Model file for the job. Use its own axes, mm. Face numbers are marked on the shaded views. Coordinates: 2 decimals unless noted, no trailing zeros. Write each loop counter-clockwise with the first axis right and the second up, starting at its lowest first coordinate (ties: lowest second). Pieces come first, ordered by that corner, then holes. Notation, with made-up numbers: M -37.75,13.5 L -11.75,13.5 A7 ccw -11.75,17.5 Z; hole C -7.75,39.25 d4. An arc over 180 degrees is marked long. Answer in a Markdown table with one row per item. Add a question column.
```python
from build123d import *
from build123d.topology import SkipClean

# Parameters (mm, degrees)
CUT_EXTRUDE_START        = -10
CUT_EXTRUDE_1_DEPTH      = 10
EXTRUDE_1_DEPTH          = 6
PATTERN_CIRCULAR_1_COUNT = 3
SKETCH_4_R               = 42.404307435
SKETCH_4_R_2             = 25.5
CUT_EXTRUDE_2_DEPTH      = 9.5
CHAMFER_START            = 14
CHAMFER_1_DEPTH          = 6


with BuildPart() as part:
    # Эскиз1 → Повернуть1 (revolve)
    with BuildSketch(Plane.XY, mode=Mode.PRIVATE) as revolve_1_sk:
        Polygon((-24, 0), (-24, 4.5), (-26, 4.5), (-26, 9.5), (-19, 9.5), (-19, 22), (-24, 22), (-24, 12.5), (-29, 12.5), (-29, 0), align=None)
    revolve(revolve_1_sk.sketch.rotate(Axis((0, 0, 0), (0, -1, 0)), 270), axis=Axis((0, 0, 0), (0, -1, 0)))

    # Эскиз2 → Вырез-Вытянуть1 (cut)
    with SkipClean():  # the faces are left unmerged after this step: merging them gives an invalid solid
        with BuildSketch(Plane(origin=(0, 0, 0), x_dir=(-1, 0, 0), z_dir=(0, -1, 0)).offset(CUT_EXTRUDE_START)):
            with BuildLine():
                ThreePointArc((24, 0), (17.8818714, -16.007456864), (2.646777063, -23.85360709))
                Line((2.646777063, -23.85360709), (5, -25.514701644))
                ThreePointArc((5, -25.514701644), (20.0748599, -16.522711642), (26, 0))
                ThreePointArc((26, 0), (25.646694472, 4.271658071), (24.596379794, 8.427223803))
                Line((24.596379794, 8.427223803), (21.981218243, 9.63462737))
                ThreePointArc((21.981218243, 9.63462737), (23.489883331, 4.921928594), (24, 0))
            make_face()
            with BuildLine():
                Line((-5, -25.514701644), (-2.646777063, -23.85360709))
                ThreePointArc((-2.646777063, -23.85360709), (-20.784609691, -12), (-21.981218243, 9.63462737))
                Line((-21.981218243, 9.63462737), (-24.596379794, 8.427223803))
                ThreePointArc((-24.596379794, 8.427223803), (-22.516660498, -13), (-5, -25.514701644))
            make_face()
            with BuildLine():
                Line((-19.596379794, 17.087477841), (-19.33444118, 14.218979719))
                ThreePointArc((-19.33444118, 14.218979719), (0, 24), (19.33444118, 14.218979719))
                Line((19.33444118, 14.218979719), (19.596379794, 17.087477841))
                ThreePointArc((19.596379794, 17.087477841), (0, 26), (-19.596379794, 17.087477841))
            make_face()
        extrude(amount=CUT_EXTRUDE_1_DEPTH, mode=Mode.SUBTRACT)

    # Эскиз3 → Бобышка-Вытянуть1 (add)
    with SkipClean():  # the faces are left unmerged after this step: merging them gives an invalid solid
        with BuildSketch(Plane(origin=(25.5, 0, 0), x_dir=(0, 0, -1), z_dir=(1, 0, 0))):
            Polygon((-11.5, 20), (11.5, 20), (11.5, 17), (-11.5, 15), align=None)
        extrude_1 = extrude(amount=-EXTRUDE_1_DEPTH)

    # Круговой массив1: Бобышка-Вытянуть1 ×3 about axis
    with SkipClean():  # the faces are left unmerged after this step: merging them gives an invalid solid
        pattern_circular_1_axis = Axis((0, 0, 0), (0, 1, 0))
        for i in range(1, PATTERN_CIRCULAR_1_COUNT):
            add(extrude_1.rotate(pattern_circular_1_axis, i * 360 / PATTERN_CIRCULAR_1_COUNT))

    # Эскиз4 → Вырез-Вытянуть2 (cut)
    with SkipClean():  # the faces are left unmerged after this step: merging them gives an invalid solid
        with BuildSketch(Plane(origin=(0, 22, 0), x_dir=(1, 0, 0), z_dir=(0, 1, 0))):
            Circle(SKETCH_4_R)
            Circle(SKETCH_4_R_2, mode=Mode.SUBTRACT)
        extrude(amount=-CUT_EXTRUDE_2_DEPTH, mode=Mode.SUBTRACT)

    # Фаска1: read off the stored shape, not the designer's step
    # Фаска1 outline → Фаска1 (cut)
    with SkipClean():  # the faces are left unmerged after this step: merging them gives an invalid solid
        with BuildSketch(Plane(origin=(0, 0, 0), x_dir=(1, 0, 0), z_dir=(0, 1, 0)).offset(CHAMFER_START)):
            with BuildLine():
                Line((-20.456443185, 12.551252218), (-20.356857991, 15.357354354))
                ThreePointArc((-20.356857991, 15.357354354), (-20.859675731, 14.667103612), (-21.33909882, 13.960403344))
                Line((-21.33909882, 13.960403344), (-20.49197936, 12.493149399))
                ThreePointArc((-20.49197936, 12.493149399), (-20.474231883, 12.522213414), (-20.456443185, 12.551252218))
            make_face()
            with BuildLine():
                ThreePointArc((-1.420514533, 25.460403344), (-2.272246462, 25.398560904), (-3.12143001, 25.308233338))
                Line((-3.12143001, 25.308233338), (-0.641481678, 23.991425578))
                ThreePointArc((-0.641481678, 23.991425578), (-0.607438987, 23.992311641), (-0.573395073, 23.993149399))
                Line((-0.573395073, 23.993149399), (-1.420514533, 25.460403344))
            make_face()
            with BuildLine():
                ThreePointArc((-20.456443185, -12.551252218), (-20.474231883, -12.522213414), (-20.49197936, -12.493149399))
                Line((-20.49197936, -12.493149399), (-21.33909882, -13.960403344))
                ThreePointArc((-21.33909882, -13.960403344), (-20.859675731, -14.667103612), (-20.356857991, -15.357354354))
                Line((-20.356857991, -15.357354354), (-20.456443185, -12.551252218))
            make_face()
            with BuildLine():
                Line((22.759613353, 11.5), (21.065374433, 11.5))
                ThreePointArc((21.065374433, 11.5), (21.08167087, 11.470098227), (21.097924862, 11.44017336))
                Line((21.097924862, 11.44017336), (23.478288, 9.950878984))
                ThreePointArc((23.478288, 9.950878984), (23.131922194, 10.731457292), (22.759613353, 11.5))
            make_face()
            with BuildLine():
                ThreePointArc((-0.573395073, -23.993149399), (-0.607438987, -23.992311641), (-0.641481678, -23.991425578))
                Line((-0.641481678, -23.991425578), (-3.12143001, -25.308233338))
                ThreePointArc((-3.12143001, -25.308233338), (-2.272246462, -25.398560904), (-1.420514533, -25.460403344))
                Line((-1.420514533, -25.460403344), (-0.573395073, -23.993149399))
            make_face()
            with BuildLine():
                ThreePointArc((22.759613353, -11.5), (23.131922194, -10.731457292), (23.478288, -9.950878984))
                Line((23.478288, -9.950878984), (21.097924862, -11.44017336))
                ThreePointArc((21.097924862, -11.44017336), (21.08167087, -11.470098227), (21.065374433, -11.5))
                Line((21.065374433, -11.5), (22.759613353, -11.5))
            make_face()
        extrude(amount=CHAMFER_1_DEPTH, mode=Mode.SUBTRACT)


solid = part.part
```
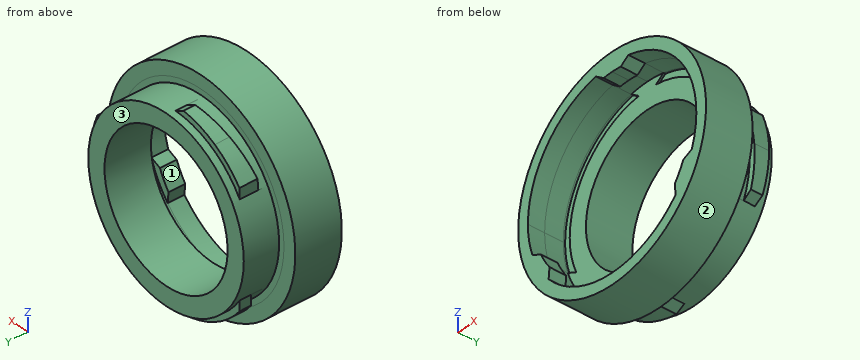
1) Slice it at A-A (x = -12). Give the cut face in (y, z), then the cut area to 3 significant figures.
2) Two-plate mould, pull along Z, no slides. Class the marked faces 1, 2 and 3: released by +Z, released by -Z, zero draft, split by the parting line, or undercut.
3) Flat gauge pins, fed straight in: pin 1 Ø4 at (x, z) = (22, -12.5) entering from +Y; pin 2 Ø1 at (y, z) = (6.5, 22.5) entering from -X; pin 3 Ø6 at (x, z) = (-16, 12.5) entering from -Y; pin 4 Ø3 at (y, z) = (15, 7) entering from -X. Where does each tip first touch, or does it go through?
4) Slice it at D-D (x = 15.5). Give the cut face in (y, z).
5) Drill centre lines: probe 1 along X at (y, z) = (17.25, 0); probe 2 along X at (y, z) = (13.5, 0); probe 3 along Y at (x, z) = (13.5, 13.5). Where is each one in solid material? Low to high.
6) Slice it at C-C (z = 23). Give the cut face in (x, y).
7) Slice it at B-B (z = 2.5). Give the cut face in (x, y), then the cut area to 3 significant figures.
Ans:
| question | item | result |
|---|---|---|
| 1 | outline | M 0,-26.4 L 12.5,-26.4 L 12.5,-20.78 L 16,-20.78 L 15.93,-22.5 L 20,-22.5 L 20,-20.78 L 22,-20.78 L 22,-14.73 L 9.5,-14.73 L 9.5,-20.78 L 10,-20.78 L 10,-23.07 L 0,-23.07 Z; M 0,23.07 L 10,23.07 L 10,20.78 L 9.5,20.78 L 9.5,14.73 L 22,14.73 L 22,20.78 L 20,20.78 L 20,22.5 L 16.07,22.5 L 16,20.78 L 12.5,20.78 L 12.5,26.4 L 0,26.4 Z |
| 1 | area | 260 mm2 |
| 2 | face 1 | undercut |
| 2 | face 2 | split by the parting line |
| 2 | face 3 | zero draft |
| 3 | pin 1 | stops at y = 22 |
| 3 | pin 2 | stops at x = -18.89 |
| 3 | pin 3 | stops at y = 9.5 |
| 3 | pin 4 | stops at x = -23.36 |
| 4 | outline | M 0,-24.51 L 12.5,-24.51 L 12.5,-18.32 L 22,-18.32 L 22,-10.99 L 9.5,-10.99 L 9.5,-18.32 L 10,-18.32 L 10,-20.87 L 0,-20.87 Z; M 0,20.87 L 10,20.87 L 10,18.32 L 9.5,18.32 L 9.5,10.99 L 22,10.99 L 22,18.32 L 12.5,18.32 L 12.5,24.51 L 0,24.51 Z |
| 5 | probe 1 | x = -24 to -19, 19 to 25.5 |
| 5 | probe 2 | x = -24 to -19, 19 to 24 |
| 5 | probe 3 | y = 9.5 to 22 |
| 6 | outline | M -17.66,0 L -12.12,0 L -12.12,10 L -6.86,10 L -6.86,9.5 L 6.86,9.5 L 6.86,10 L 12.12,10 L 12.12,0 L 17.66,0 L 17.66,12.5 L 6.86,12.5 L 6.86,22 L -6.86,22 L -6.86,20 L -11.01,20 L -11.01,16.17 L -6.86,16.48 L -6.86,12.5 L -17.66,12.5 Z |
| 7 | outline | M -28.89,0 L -25.88,0 L -25.88,10 L -23.87,10 L -23.87,9.5 L -18.83,9.5 L -18.83,22 L -23.87,22 L -23.87,12.5 L -28.89,12.5 Z; M 18.83,9.5 L 23.87,9.5 L 23.87,10 L 25.88,10 L 25.88,0 L 28.89,0 L 28.89,12.5 L 23.87,12.5 L 23.87,15.78 L 25.38,15.78 L 25.38,20 L 23.87,20 L 23.87,22 L 18.83,22 Z |
| 7 | area | 218 mm2 |
